```python
from build123d import *

# Parameters (mm, degrees)
SKETCH1_R           = 3
SKETCH1_W           = 7.8
SKETCH1_H           = 4.7
SKETCH1_R_2         = 8.95
BOSS_EXTRUDE1_DEPTH = 30.6
CUT_EXTRUDE1_DEPTH  = 26.1
FILETE1_R           = 1.5


with BuildPart() as part:
    # Sketch1 → Boss-Extrude1 (new body)
    with BuildSketch(Plane.XY):
        with BuildLine():
            ThreePointArc((77.466015174, -30.925650144), (98.9, 0), (77.466015174, 30.925650144))
            Line((77.466015174, 30.925650144), (19.70985088, 52.577031851))
            ThreePointArc((19.70985088, 52.577031851), (-56.15, 0), (19.70985088, -52.577031851))
            Line((19.70985088, -52.577031851), (77.466015174, -30.925650144))
        make_face()
        with BuildLine():
            Line((63.45, 15.95), (66.35, 15.95))
            ThreePointArc((66.35, 15.95), (82.3, 0), (66.35, -15.95))
            Line((66.35, -15.95), (63.45, -15.95))
            ThreePointArc((63.45, -15.95), (47.5, 0), (63.45, 15.95))
        make_face(mode=Mode.SUBTRACT)
        with Locations((30.55, 0)):
            Circle(SKETCH1_R, mode=Mode.SUBTRACT)
        with Locations((82.211647497, -17.5)):
            Rectangle(SKETCH1_W, SKETCH1_H, mode=Mode.SUBTRACT)
        with Locations((82.211647497, 17.5)):
            Rectangle(SKETCH1_W, SKETCH1_H, mode=Mode.SUBTRACT)
        with Locations((47.211647497, 17.5)):
            Rectangle(SKETCH1_W, SKETCH1_H, mode=Mode.SUBTRACT)
        with Locations((47.211647497, -17.5)):
            Rectangle(SKETCH1_W, SKETCH1_H, mode=Mode.SUBTRACT)
        Circle(SKETCH1_R_2, mode=Mode.SUBTRACT)
        with Locations((0, 30.55)):
            Circle(SKETCH1_R, mode=Mode.SUBTRACT)
        with Locations((0, -30.55)):
            Circle(SKETCH1_R, mode=Mode.SUBTRACT)
        with Locations((-30.55, 0)):
            Circle(SKETCH1_R, mode=Mode.SUBTRACT)
    extrude(amount=BOSS_EXTRUDE1_DEPTH)

    # Sketch2 → Cut-Extrude1 (cut)
    with BuildSketch(Plane.XY.offset(30.6)):
        with BuildLine():
            Line((77.009687371, 29.70837247), (19.253523077, 51.359754177))
            ThreePointArc((19.253523077, 51.359754177), (-54.85, 0), (19.253523077, -51.359754177))
            Line((19.253523077, -51.359754177), (77.009687371, -29.70837247))
            ThreePointArc((77.009687371, -29.70837247), (97.6, 0), (77.009687371, 29.70837247))
        make_face()
    extrude(amount=-CUT_EXTRUDE1_DEPTH, mode=Mode.SUBTRACT)

    # Filete1
    filete1_edges = [part.edges().sort_by_distance(p)[0] for p in [
        (51.111647497, -19.85, 2.25),
        (51.111647497, -15.15, 2.25),
        (86.111647497, -19.85, 2.25),
        (86.111647497, -15.15, 2.25),
        (51.111647497, 15.15, 2.25),
        (51.111647497, 19.85, 2.25),
        (43.311647497, -15.15, 2.25),
        (43.311647497, -19.85, 2.25),
        (78.311647497, -15.15, 2.25),
        (78.311647497, -19.85, 2.25),
        (86.111647497, 15.15, 2.25),
        (86.111647497, 19.85, 2.25),
        (78.311647497, 19.85, 2.25),
        (78.311647497, 15.15, 2.25),
        (43.311647497, 19.85, 2.25),
        (43.311647497, 15.15, 2.25),
    ]]
    fillet(filete1_edges, radius=FILETE1_R)


solid = part.part
```
Verification items for the finished model (mm, model axes). A direction names the side the tool comes from. Coordinates: 2 decimals unless noted, no trailing zeros. Order: outer loops, then holes, each group sorted by start corner. A loop starts at its lowest first (then second) coordinate and runs counter-clockwise, first axis right, second up. Notation, with made-up numbers: (-6.75, -34) -> (11.25, -34) arc R25 cw to (11.25, -10) -> close; hole circle Ø11 at (30.25, 2). An arc over 180 degrees is marked (long way). Put each result on its own line as item: value. Start each with the question number.
1) Release check for a two-part mould opening along Y. For faces 1 (the flat face through (47, 19.85, 2)), 2 (the flat face through (48.99, 41.6, 15.09)), 3 (the cylindrical face through (98.895, -0.56, 15.086)) record: pulls with the +Y half, pulls with the -Y half, needs draft (parallel to the pull), parting line crosses it, or undercut.
2) Cross-section at B-B (x = 0). Enter the section's corners in (y, z).
3) Cross-section at A-A (y = 0). Enter the section's corners in (x, z).
4) Go/stop test with flat-tipped pins: pin 1 (1.9 mm diameter, centred on y = 17.5, z = 2.5, fed in from +X); pin 2 (4 mm diameter, centred on y = 30.5, z = 19, fed in from +X); pin 3 (0.9 mm diameter, centred on x = 64, z = 1.5, fed in from +Y). Record where each tip stops, or that it passes through.
5) Cross-section at C-C (z = 28.5). Enter the section's corners in (x, y), plus the area to 3 significant figures.
6) Tool access check on faces 4 (the flat face through (82, 19.85, 2)), 5 (the flat face through (9.5, 54.3, 30.6)), 6 (the flat face through (47.727, -40.686, 17.733)). Record the directions out of +Z, -Z, +X, -X, +Y, -Y that give a thin tool (end or side, any length) a straight path to the whole face; none if there is none.
7) Material ranges on L1, parallel to Y at x = 0, z = 2; L2, parallel to X at y = 0, z = 1; L3, parallel to X at y = -16, z = 4, recorded low to high.
8) Cross-section at D-D (x = 75). Enter the section's corners in (y, z), plus the area to 3 significant figures.
Geometry check:
1. face 1: undercut
1. face 2: pulls with the +Y half
1. face 3: parting line crosses it
2. outline: (-56.15, 0) -> (-33.55, 0) -> (-33.55, 4.5) -> (-54.85, 4.5) -> (-54.85, 30.6) -> (-56.15, 30.6) -> close; (-27.55, 0) -> (-8.95, 0) -> (-8.95, 4.5) -> (-27.55, 4.5) -> close; (8.95, 0) -> (27.55, 0) -> (27.55, 4.5) -> (8.95, 4.5) -> close; (33.55, 0) -> (56.15, 0) -> (56.15, 30.6) -> (54.85, 30.6) -> (54.85, 4.5) -> (33.55, 4.5) -> close
3. outline: (-56.15, 0) -> (-33.55, 0) -> (-33.55, 4.5) -> (-54.85, 4.5) -> (-54.85, 30.6) -> (-56.15, 30.6) -> close; (-27.55, 0) -> (-8.95, 0) -> (-8.95, 4.5) -> (-27.55, 4.5) -> close; (8.95, 0) -> (27.55, 0) -> (27.55, 4.5) -> (8.95, 4.5) -> close; (33.55, 0) -> (47.5, 0) -> (47.5, 4.5) -> (33.55, 4.5) -> close; (82.3, 0) -> (98.9, 0) -> (98.9, 30.6) -> (97.6, 30.6) -> (97.6, 4.5) -> (82.3, 4.5) -> close
4. pin 1: stops at x = 94.45
4. pin 2: stops at x = 82.56
4. pin 3: stops at y = 36.14
5. outline: (19.71, -52.58) -> (77.47, -30.93) arc R33.03 ccw to (77.47, 30.93) -> (19.71, 52.58) arc R56.15 ccw (long way) to start; hole (19.25, -51.36) -> (77.01, -29.71) arc R31.73 ccw to (77.01, 29.71) -> (19.25, 51.36) arc R54.85 ccw (long way) to start
5. area: 541 mm^2
6. face 4: +Z, -Z
6. face 5: +Z, +X, -X, +Y, -Y
6. face 6: +Z
7. L1: y = -56.15 to -33.55, -27.55 to -8.95, 8.95 to 27.55, 33.55 to 56.15
7. L2: x = -56.15 to -33.55, -27.55 to -8.95, 8.95 to 27.55, 33.55 to 47.5, 82.3 to 98.9
7. L3: x = -53.82 to 43.46, 50.96 to 78.46, 85.96 to 94.77
8. outline: (-31.85, 0) -> (-13.4, 0) -> (-13.4, 4.5) -> (-30.46, 4.5) -> (-30.46, 30.6) -> (-31.85, 30.6) -> close; (13.4, 0) -> (31.85, 0) -> (31.85, 30.6) -> (30.46, 30.6) -> (30.46, 4.5) -> (13.4, 4.5) -> close
8. area: 239 mm^2
